Job drawing, mm, ordinate dimensions from the low corner. One solid piece. A direction names the side the tool comes from. Round coordinates to 2 decimals unless told otherwise and drop trailing zeros. Order: outer loops, then holes, each group sorted by start corner. A loop starts at its lowest first (then second) coordinate and runs counter-clockwise, first axis right, second up. Notation, with made-up numbers: (48, 85) -> (96, 85) arc R18 ccw to (96, 111) -> close; hole circle Ø6 at (29.25, 68). An arc over 180 degrees is marked (long way). Write item = value, one per line.
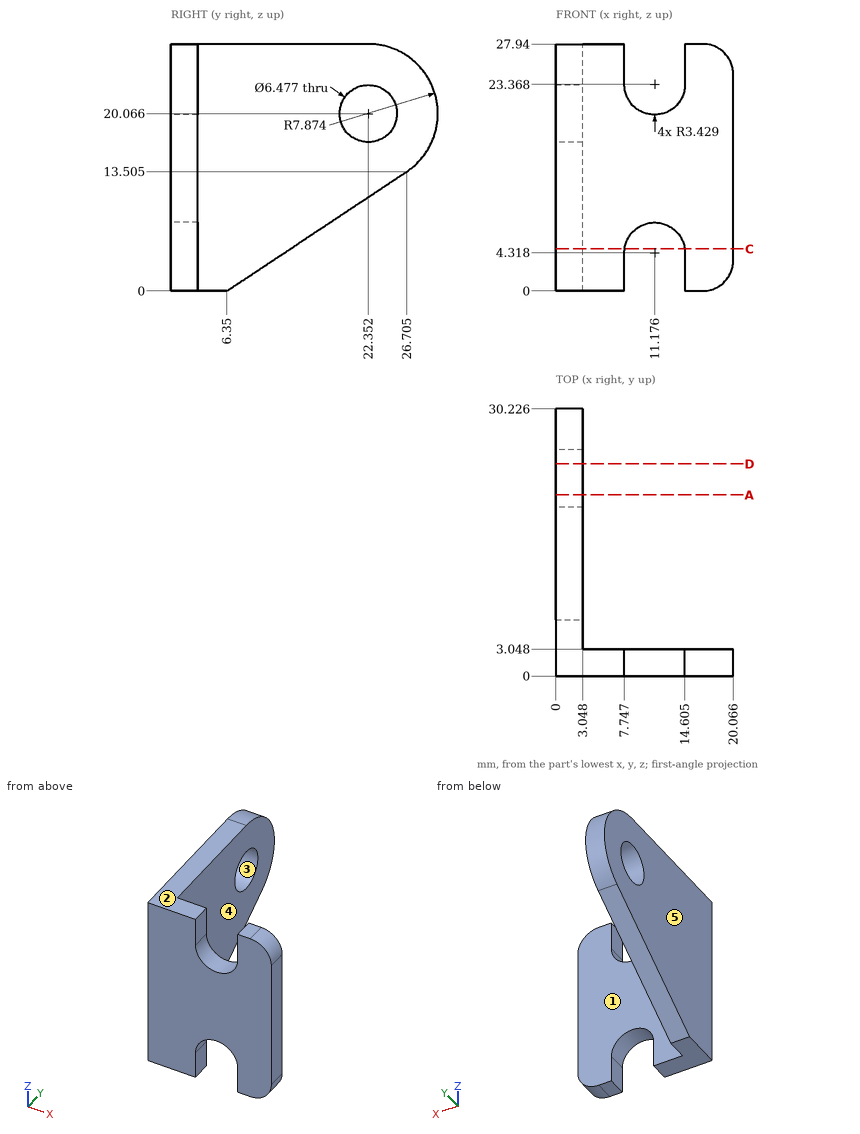
Q1. Which spindle directions (+Z, -Z, +X, -X, +Y, -Y) get a long thin tool onto all of the face, cutting with end or side? Do the marked faces 4 and 5. Say none if no direction does.
Check values:
face_4 = +Z, -Z, +X, +Y
face_5 = +Z, -Z, -X, +Y, -Y
Q2. Probe probe 1 along Y at (x, z) = (18.5, 5); probe 2 along Z at (x, y) = (1.25, 13.5). List the from-to ranges inside material, lowest first.
Check values:
probe_1 = 0 to 3.05
probe_2 = 4.74 to 27.94
Q3. Cut at C-C, the plane z = 4.75. List the corners of the cut face in (x, y).
Check values:
outline = (0, 0) -> (7.77, 0) -> (7.77, 3.05) -> (3.05, 3.05) -> (3.05, 13.51) -> (0, 13.51) -> close; (14.58, 0) -> (20.07, 0) -> (20.07, 3.05) -> (14.58, 3.05) -> close
Q4. Cut at A-A, the plane y = 20.5. List the corners of the cut face in (x, z).
Check values:
outline = (0, 9.39) -> (3.05, 9.39) -> (3.05, 17.41) -> (0, 17.41) -> close; (0, 22.72) -> (3.05, 22.72) -> (3.05, 27.94) -> (0, 27.94) -> close
Q5. Cut at D-D, the plane y = 24. List the corners of the cut face in (x, z).
Check values:
outline = (0, 11.71) -> (3.05, 11.71) -> (3.05, 17.28) -> (0, 17.28) -> close; (0, 22.85) -> (3.05, 22.85) -> (3.05, 27.77) -> (0, 27.77) -> close
Q6. Mould opens along Y. For the marked faces 1, 2 and 3 say: released by +Y, released by -Y, zero draft, split by the parting line, or undercut.
Check values:
face_1 = released by +Y
face_2 = zero draft
face_3 = undercut
Q7. Flat gauge pins, fed straight in: pin 1 (6 mm diameter, centred on x = 7.5, y = 23.5, fed in from -Z); pin 2 (4 mm diameter, centred on y = 24, z = 12.5, fed in from +X); pin 3 (1.5 mm diameter, centred on y = 2, z = 25.5, fed in from +X); pin 4 (4 mm diameter, centred on x = 5.5, z = 7.5, fed in from +Y). Where does each tip first touch, or does it go through?
Check values:
pin_1 = through
pin_2 = 3.05
pin_3 = 20.06
pin_4 = 3.05
